Autodesk Inventor part; units mm, degrees
ref_plane "YZ Plane" through (0, 0, 0) normal (1, 0, 0) x (0, 1, 0)
ref_plane "XZ Plane" through (0, 0, 0) normal (0, 1, 0) x (-1, 0, 0)
ref_plane "XY Plane" through (0, 0, 0) normal (0, 0, 1) x (1, 0, 0)
sketch "Sketch7" plane through (0, 0, 0) normal (0, 1, 0) x (-1, 0, 0)
  point P0 (0, 0)
sketch "Sketch8" plane through (0, 0, 0) normal (0, 1, 0) x (-1, 0, 0)
  line L0 (0, 0) -> (-29, 0)
  line L1 (-29, 0) -> (-29, -29)
  line L2 (-29, -29) -> (0, -29)
  line L3 (0, -29) -> (0, 0)
  line L4 (-2, -27) -> (-27, -27)
  line L5 (-27, -27) -> (-27, -2)
  line L6 (-27, -2) -> (-2, -2)
  line L7 (-2, -2) -> (-2, -27)
  dimension "d25" = 29
  dimension "d26" = 29
  dimension "d38" = 2
extrude "Extrusion5" add sketch "Sketch8" along normal blind 30 contours L3 L2 L1 L0 | L4 L5 L6 L7
sketch "Sketch11" plane through (0, 30, 0) normal (0, 1, 0) x (1, 0, 0)
  line L0 (0, 0) -> (29, 0)
  line L1 (29, 0) -> (29, 29)
  line L2 (29, 29) -> (0, 29)
  line L3 (0, 29) -> (0, 0)
  line L4 (2, 27) -> (27, 27)
  line L5 (27, 27) -> (27, 2)
  line L6 (27, 2) -> (2, 2)
  line L7 (2, 2) -> (2, 27)
  dimension "d39" = 2
extrude "Extrusion8" cut sketch "Sketch11" against normal blind 28 contours L4 L5 L6 L7
equation "\"BendRadius\" = Thickness"
equation "\"BendReliefWidth\" = Thickness"
equation "\"BendReliefDepth\" = 0.5 * Thickness"
equation "\"CornerReliefSize\" = 4 * Thickness"
equation "\"MinimumRemnant\" = 2 * Thickness"
equation "\"TransitionRadius\" = BendRadius"
equation "\"JacobiRadiusSize\" = Thickness"
equation "\"GapSize\" = Thickness"
properties part number "waterBallonHolderv2"
Read the model definition and answer for the solid it produces. Units are mm, in the model's axes. A direction names the side the tool comes from. Give positions to 0.01 mm unless a question says otherwise; leave off trailing zeros. Write each loop counter-clockwise with the first axis right and the second up, starting at its lowest first coordinate (ties: lowest second). Pieces come first, ordered by that corner, then holes. Notation, with made-up numbers: (25, -25.75) - (70, -25.75) arc R28 cw to (70, 4.25) - close; hole circle Ø4 at (-2, 15). An arc over 180 degrees is marked (long way). Use CSV: the item, a comma, the result in double quotes. Start each with the question number.
(1) Consider line 1 along Z through (x, y) = (18.25, 6.5); line 2 along X through (y, z) = (14.5, -3.25); line 3 along Y through (x, z) = (6, -7.5). Determine where each line is inside the solid, lowest interval first.
(2) For faces 5 (the flat face through (29, 15, -14)), 6 (the flat face through (27, 16, -15)), determine the directions among +Z, -Z, +X, -X, +Y, -Y from which every point of the face is accessible in a straight line to the end or side of a thin tool.
(3) Find section B-B (z = -12.25). Give the vertices of the cut face in (x, y), plus the area to 3 significant figures.
(4) Find section C-C (x = 18.25). Give the vertices of the cut face in (y, z), plus the area to 3 significant figures.
(5) Determine the mould class of faces 1 (the flat face through (14, 15, 0)), 2 (the flat face through (15, 15, -29)), 3 (the flat face through (14, 2, -15)), 4 (the flat face through (0, 15, -15)) for opening direction Z: +Z half, -Z half, draft (parallel to the pull), parting line (faces both ways), or undercut.
(6) Given P1, Ø2, axis at x = 17, z = -5.5, coming from the +Y side, flat-ended and moving along its own axis, determine where the tip first touches the part or whether it passes through.
(7) Find section A-A (y = 16). Give the vertices of the cut face in (x, z).
Findings below:
1,line 1,"-29 to -27, -2 to 0"
1,line 2,"0 to 2, 27 to 29"
1,line 3,"0 to 2"
2,face 5,"+Z, -Z, +X, +Y, -Y"
2,face 6,"+Y"
3,outline,"(0, 0) - (29, 0) - (29, 30) - (27, 30) - (27, 2) - (2, 2) - (2, 30) - (0, 30) - close"
3,area,"170 mm2"
4,outline,"(0, -29) - (30, -29) - (30, -27) - (2, -27) - (2, -2) - (30, -2) - (30, 0) - (0, 0) - close"
4,area,"170 mm2"
5,face 1,"+Z half"
5,face 2,"-Z half"
5,face 3,"undercut"
5,face 4,"draft"
6,P1,"y = 2"
7,outline,"(0, -29) - (29, -29) - (29, 0) - (0, 0) - close; hole (2, -27) - (27, -27) - (27, -2) - (2, -2) - close"
